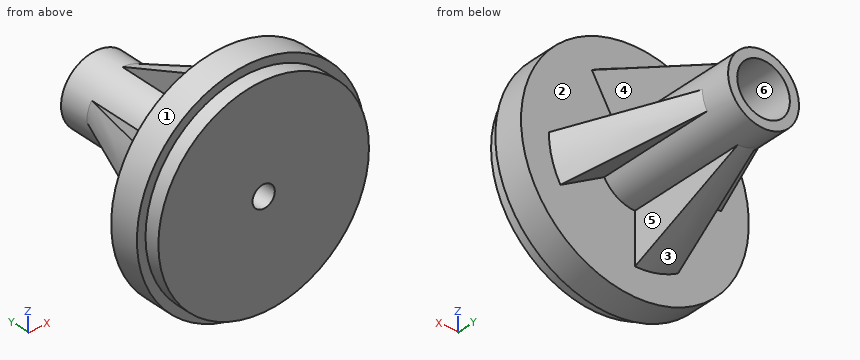
from build123d import *

# Parameters (mm, degrees)
SKETCH_1_R          = 10.4
EXTRUDE_1_DEPTH     = 1.5
SKETCH_2_R          = 11.25
EXTRUDE_2_DEPTH     = 3
SKETCH_3_R          = 3.5
SKETCH_3_R_2        = 2.6
EXTRUDE_3_DEPTH     = 15
SKETCH_3_4_R        = 1.1
CUT_EXTRUDE_2_DEPTH = 4.5
REVOLVE_3_ANGLE     = 30
REVOLVE_4_ANGLE     = 30


with BuildPart() as part:
    # 草图1 → 凸台-拉伸1 (new body)
    with BuildSketch(Plane(origin=(0, 0, 0), x_dir=(1, 0, 0), z_dir=(0, 1, 0))):
        with Locations(Location((0, 0, 0), (0, 0, 270))):
            Circle(SKETCH_1_R)
    extrude(amount=EXTRUDE_1_DEPTH)

    # 草图2 → 凸台-拉伸2 (add)
    with BuildSketch(Plane(origin=(0, 1.5, 0), x_dir=(1, 0, 0), z_dir=(0, 1, 0))):
        with Locations(Location((0, 0, 0), (0, 0, 270))):
            Circle(SKETCH_2_R)
    extrude(amount=EXTRUDE_2_DEPTH)

    # 草图3 → 凸台-拉伸3 (add)
    with BuildSketch(Plane(origin=(0, 4.5, 0), x_dir=(1, 0, 0), z_dir=(0, 1, 0))):
        with Locations(Location((0, 0, 0), (0, 0, 270))):
            Circle(SKETCH_3_R)
        with Locations(Location((0, 0, 0), (0, 0, 270))):
            Circle(SKETCH_3_R_2, mode=Mode.SUBTRACT)
    extrude(amount=EXTRUDE_3_DEPTH)

    # 草图3<4> → 切除-拉伸2 (cut)
    with BuildSketch(Plane(origin=(0, 4.5, 0), x_dir=(1, 0, 0), z_dir=(0, 1, 0))):
        with Locations(Location((0, 0, 0), (0, 0, 270))):
            Circle(SKETCH_3_4_R)
    extrude(amount=-CUT_EXTRUDE_2_DEPTH, mode=Mode.SUBTRACT)

    # 草图6 → 旋转3 (revolve)
    with BuildSketch(Plane(origin=(0, 0, 0), x_dir=(0, 0, -1), z_dir=(1, 0, 0))):
        Polygon((3.5, 4.5), (3.5, 16.5), (8.5, 4.5), align=None)
        Polygon((-8.5, 4.5), (-3.5, 4.5), (-3.5, 16.5), align=None)
    revolve(axis=Axis((0, 0, 0), (0, 1, 0)), revolution_arc=REVOLVE_3_ANGLE)

    # 草图9 → 旋转4 (revolve)
    with BuildSketch(Plane.XY):
        Polygon((3.5, 4.5), (8.5, 4.5), (3.5, 16.5), align=None)
        Polygon((-8.5, 4.5), (-3.5, 16.5), (-3.5, 4.5), align=None)
    revolve(axis=Axis((0, 0, 0), (0, 1, 0)), revolution_arc=REVOLVE_4_ANGLE)


solid = part.part
Design review of the part built by this model. Coordinates are the model's own, in mm. Face numbers are marked on the shaded views. A direction names the side the tool comes from. Coordinates: 2 decimals unless noted, no trailing zeros. Order: outer loops, then holes, each group sorted by start corner. A loop starts at its lowest first (then second) coordinate and runs counter-clockwise, first axis right, second up. Notation, with made-up numbers: (82, -28) - (105, -28) arc R29 ccw to (105, 11) - close; hole circle Ø9 at (33.5, -4). An arc over 180 degrees is marked (long way). Put each result on its own line as item: value.
1) Tool access review of the marked faces 1 and 2: name each direction out of +Z, -Z, +X, -X, +Y, -Y from which nothing blocks a thin tool from reaching the whole face with its end or side.
Response values:
face 1: +Y, -Y
face 2: +Y
2) Take a section at C-C, the plane y = 17.5. Give the boundary of the cut face in (x, z).
Response values:
outline: circle Ø7 at (0, 0); hole circle Ø5.2 at (0, 0)
3) Wall thickness on L1, parallel to X at y = 3.55, z = 0; L2, parallel to X at y = 1.2, z = 0; L3, parallel to Y at x = 9, z = -3.75: over which ranges is each line inside the solid? List them lowest first. Write a range as from..to.
Response values:
L1: x = -11.25..-1.1, 1.1..11.25
L2: x = -10.4..-1.1, 1.1..10.4
L3: y = 0..4.5
4) Insertion check: P1, Ø1, axis at x = -3.5, y = 17, coming from the -Z side; P2, Ø4, axis at x = 6, y = 13.5, coming from the +Z side; P3, Ø3, axis at y = 13, z = 6, coming from the +X side. Each pin has a flat end and moves straight along its axis. Give the tip position at first contact, or say it passes through.
Response values:
P1: stops at z = -1.8
P2: stops at z = 0
P3: stops at x = 2.4
5) Take a section at A-A, the plane y = 14. Give the boundary of the cut face in (x, z).
Response values:
outline: (-4.54, 0) - (-3.5, 0) arc R3.5 ccw to (-1.75, -3.03) - (-2.27, -3.93) arc R4.54 ccw to (0, -4.54) - (0, -3.5) arc R3.5 ccw to (3.03, -1.75) - (3.93, -2.27) arc R4.54 ccw to (4.54, 0) - (3.5, 0) arc R3.5 ccw to (1.75, 3.03) - (2.27, 3.93) arc R4.54 ccw to (0, 4.54) - (0, 3.5) arc R3.5 ccw to (-3.03, 1.75) - (-3.93, 2.27) arc R4.54 ccw to start; hole circle Ø5.2 at (0, 0)
6) Take a section at B-B, the plane x = 9. Give the boundary of the cut face in (y, z).
Response values:
outline: (0, -5.21) - (1.5, -5.21) - (1.5, -6.75) - (4.5, -6.75) - (4.5, 6.75) - (1.5, 6.75) - (1.5, 5.21) - (0, 5.21) - close
7) The part is to be moulded in two halves that separate along Z. For the marked faces 3, 4, 5 and 6, say which applies: released by +Z, released by -Z, zero draft, split by the parting line, or undercut.
Response values:
face 3: released by -Z
face 4: undercut
face 5: zero draft
face 6: undercut
